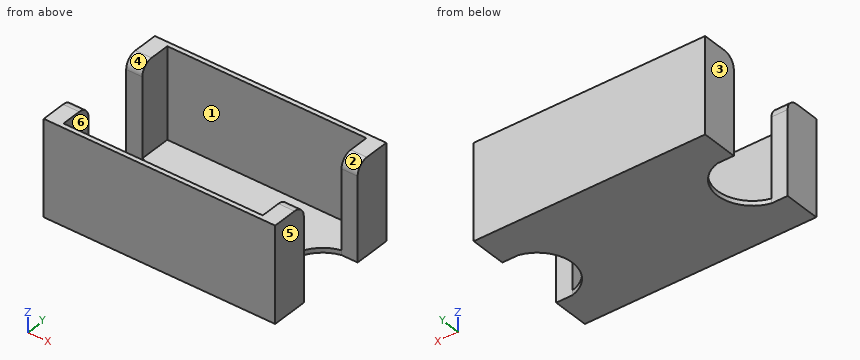
from build123d import *

# Parameters (mm, degrees)
SKETCH029_W          = 79
SKETCH029_H          = 48.2
SKETCH029_W_2        = 68
SKETCH029_H_2        = 45
PAD015_DEPTH         = 31
SKETCH091_W          = 79
SKETCH091_H          = 48.2
PAD054_DEPTH         = 1.6
POCKET037_DEPTH      = 1.601
POCKET037_DEPTH_BACK = 31.001
FILLET009_R          = 4


with BuildPart() as part:
    # Sketch029 → Pad015 (new body)
    with BuildSketch(Plane.XY):
        Rectangle(SKETCH029_W, SKETCH029_H)
        Rectangle(SKETCH029_W_2, SKETCH029_H_2, mode=Mode.SUBTRACT)
    extrude(amount=PAD015_DEPTH)

    # Sketch091 → Pad054 (join)
    with BuildSketch(Plane.XY):
        Rectangle(SKETCH091_W, SKETCH091_H)
    extrude(amount=-PAD054_DEPTH)

    # Sketch030 → Pocket037 (cut, two sides)
    with BuildSketch(Plane.XY) as pocket037_sk:
        with BuildLine():
            ThreePointArc((-34, -11.680646), (-24.75, 0), (-34, 11.680646))
            Line((-34, 11.680646), (-39.5, 11.680646))
            Line((-39.5, 11.680646), (-39.5, -11.680646))
            Line((-34, -11.680646), (-39.5, -11.680646))
        make_face()
        with BuildLine():
            ThreePointArc((34, 11.680646), (24.75, 0), (34, -11.680646))
            Line((34, -11.680646), (39.5, -11.680646))
            Line((39.5, 11.680646), (39.5, -11.680646))
            Line((34, 11.680646), (39.5, 11.680646))
        make_face()
    extrude(amount=-POCKET037_DEPTH, mode=Mode.SUBTRACT)
    extrude(pocket037_sk.sketch, amount=POCKET037_DEPTH_BACK, mode=Mode.SUBTRACT)

    # Fillet009
    fillet009_edges = [part.edges().sort_by_distance(p)[0] for p in [
        (36.75, 11.680646, 31),
        (36.75, -11.680646, 31),
        (-36.75, 11.680646, 31),
        (-36.75, -11.680646, 31),
    ]]
    fillet(fillet009_edges, radius=FILLET009_R)


solid = part.part
Can you work these out from the model? Positions are in its coordinate system, mm. Face numbers are marked on the shaded views. A direction names the side the tool comes from. Give positions to 0.01 mm unless a question says otherwise; leave off trailing zeros. Loops run counter-clockwise (first coordinate to the right, second up) from the corner with the lowest first, then second, coordinate; pieces in that order, holes last. Notation, with made-up numbers: M -20.75,57 L 30.25,57 A12 ccw 30.25,72 Z; hole C 65.25,13.25 d11. An arc over 180 degrees is marked long. One line per item, written item: value.
1) Thinking about a two-plate mould opening in X: for the marked faces 1, 2 and 3, which applies, +X half, -X half, draft (parallel to the pull), parting line (faces both ways), or undercut?
Geometry check:
face 1: undercut
face 2: draft
face 3: -X half
2) Imagine slicing it at B-B on x = 29. Write out the boundary of the cut face in (y, z), and give its area (3 significant figures).
Geometry check:
outline: M -24.1,-1.6 L -9.16,-1.6 L -9.16,0 L -22.5,0 L -22.5,31 L -24.1,31 Z; M 9.16,-1.6 L 24.1,-1.6 L 24.1,31 L 22.5,31 L 22.5,0 L 9.16,0 Z
area: 147 mm²
3) Imagine slicing it at A-A on z = 3.5. Write out the boundary of the cut face in (x, y).
Geometry check:
outline: M -39.5,-24.1 L 39.5,-24.1 L 39.5,-11.68 L 34,-11.68 L 34,-22.5 L -34,-22.5 L -34,-11.68 L -39.5,-11.68 Z; M -39.5,11.68 L -34,11.68 L -34,22.5 L 34,22.5 L 34,11.68 L 39.5,11.68 L 39.5,24.1 L -39.5,24.1 Z
4) Imagine slicing it at C-C on y = 20. Write out the boundary of the cut face in (x, z).
Geometry check:
outline: M -39.5,-1.6 L 39.5,-1.6 L 39.5,31 L 34,31 L 34,0 L -34,0 L -34,31 L -39.5,31 Z
5) On a 3-axis mill with a long thin cutter (end or side, diameter ignored), from which of +Z, -Z, +X, -X, +Y, -Y can I reach the whole of each face in a straight line? I mean the marked faces 4, 5 and 6. Say none if no direction works.
Geometry check:
face 4: +Z, +X, -X
face 5: +Z, -Z, +X, +Y, -Y
face 6: +Z
6) Imagine slicing it at D-D on x = -17.5. Write out the boundary of the cut face in (y, z), and give its area (3 significant figures).
Geometry check:
outline: M -24.1,-1.6 L 24.1,-1.6 L 24.1,31 L 22.5,31 L 22.5,0 L -22.5,0 L -22.5,31 L -24.1,31 Z
area: 176 mm²
7) Please list where these lines run through material, in increasing order: line 1 (Y direction, x = -35, z = 22); line 2 (X direction, y = -21, z = 29); line 3 (Y direction, x = 18.5, z = 5).
Geometry check:
line 1: y = -24.1 to -11.68, 11.68 to 24.1
line 2: x = -39.5 to -34, 34 to 39.5
line 3: y = -24.1 to -22.5, 22.5 to 24.1
